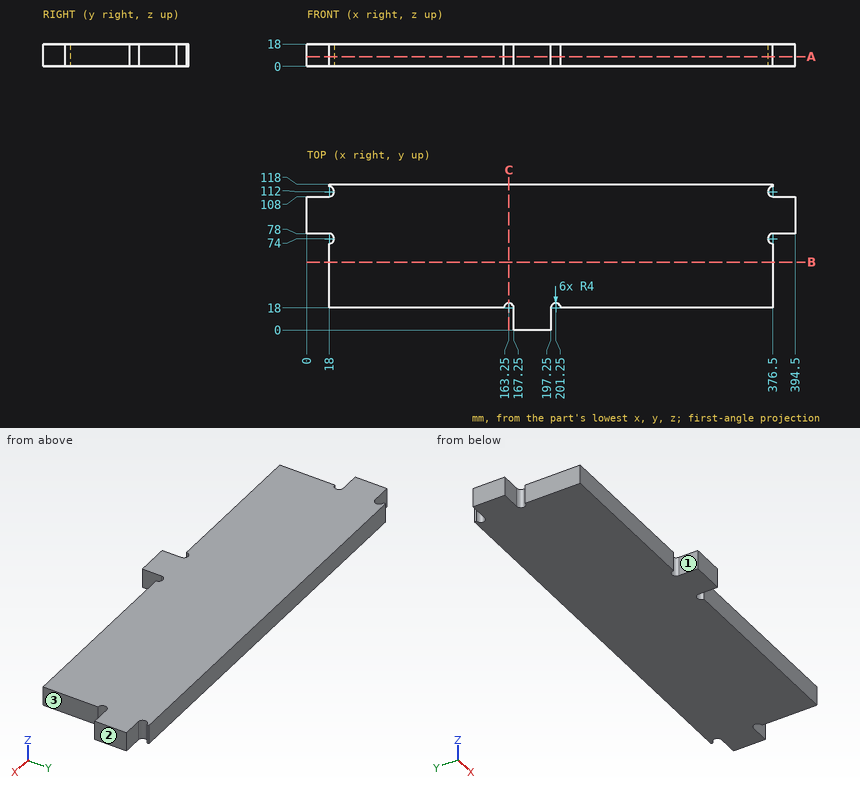
The drawing under review shows one solid part. Ordinate dimensions are in mm from its lowest x, y, z. A direction names the side the tool comes from. Round coordinates to 2 decimals unless told otherwise and drop trailing zeros. Loops run counter-clockwise (first coordinate to the right, second up) from the corner with the lowest first, then second, coordinate; pieces in that order, holes last. Notation, with made-up numbers: (68.5, -25.75) - (126.5, -25.75) arc R20 cw to (126.5, -18.75) - close; hole circle Ø8 at (29, 49.5). An arc over 180 degrees is marked (long way). Put each result on its own line as item: value. Start each with the question number.
1. Insertion check: P1, Ø5.5, axis at x = 13, z = 11.5, coming from the -Y side; P2, Ø9, axis at y = 11.5, z = 10.5, coming from the -X side; P3, Ø8, axis at x = 151, z = 6, coming from the -Y side. Each pin has a flat end and moves straight along its axis. Give the tip position at first contact, or say it passes through.
2. Consider section C-C on x = 163.25. State the section outline as (y, z) points, plus the area to 3 significant figures.
3. Consider section A-A on z = 7.75. State the section outline as (x, y) points.
4. Consider section B-B on y = 55. State the section outline as (x, z) points, plus the area to 3 significant figures.
5. For probe 1 along X at (y, z) = (9, 8.25); probe 2 along Y at (x, z) = (261, 4.5); probe 3 along X at (y, z) = (59, 2), list the stretches that pass through material, from the lowest coordinate up. Write a range as [from, to].
6. For the marked faces 1, 2 and 3, list the 3-axis set-ups (+Z, -Z, +X, -X, +Y, -Y) from which the entire face can be reached by the end or side of a thin tool; tool diameter is ignored.
Result sheet:
1. P1: y = 78
1. P2: x = 167.25
1. P3: y = 18
2. outline: (22, 0) - (118, 0) - (118, 18) - (22, 18) - close
2. area: 1,730 mm^2
3. outline: (0, 78) - (18, 78) arc R4 cw to (18, 70) - (18, 18) - (159.25, 18) arc R4 cw to (167.25, 18) - (167.25, 0) - (197.25, 0) - (197.25, 18) arc R4 cw to (205.25, 18) - (376.5, 18) - (376.5, 70) arc R4 cw to (376.5, 78) - (394.5, 78) - (394.5, 108) - (376.5, 108) arc R4 cw to (376.5, 116) - (376.5, 118) - (18, 118) - (18, 116) arc R4 cw to (18, 108) - (0, 108) - close
4. outline: (18, 0) - (376.5, 0) - (376.5, 18) - (18, 18) - close
4. area: 6,450 mm^2
5. probe 1: [167.25, 197.25]
5. probe 2: [18, 118]
5. probe 3: [18, 376.5]
6. face 1: +Z, -Z, -X, -Y
6. face 2: +Z, -Z, +X, +Y, -Y
6. face 3: +Z, -Z, +X, -Y
